Source: CAD feature listing. Evaluate the final solid. Frame: model axes, mm. Face numbers are marked on the shaded views. Give positions to 0.01 mm unless a question says otherwise; leave off trailing zeros. Order: outer loops, then holes, each group sorted by start corner. A loop starts at its lowest first (then second) coordinate and runs counter-clockwise, first axis right, second up. Notation, with made-up numbers: (48.5, -18.75) -> (65.5, -18.75) arc R13 cw to (65.5, -6.75) -> close; hole circle Ø1 at (-19.5, 17). An arc over 180 degrees is marked (long way). Use CSV: the item, a comma, the result in double quotes.
```python
from build123d import *

# Parameters (mm, degrees)
F1_DEPTH = 40.2336
F0_R     = 10.16
F2_DEPTH = 15.7734
F3_R     = 3.302


with BuildPart() as f1:
    # F0 (on Front) → F1 (new body)
    with BuildSketch(Plane.XZ):
        with BuildLine():
            ThreePointArc((9.5121844836, 26.9452959039), (4.8253908933, 28.1646272428), (0, 28.575))
            Line((0, 28.575), (9.5121844836, 26.9452959039))
        make_face()
        with BuildLine():
            Line((9.5121844836, -26.9452959039), (0, -28.575))
            ThreePointArc((0, -28.575), (4.8253908933, -28.1646272428), (9.5121844836, -26.9452959039))
        make_face()
        with BuildLine():
            Line((9.5121844836, 26.9452959039), (0, 28.575))
            ThreePointArc((0, 28.575), (-28.575, 0), (0, -28.575))
            Line((0, -28.575), (9.5121844836, -26.9452959039))
            ThreePointArc((9.5121844836, -26.9452959039), (23.3274655355, -16.5033322905), (28.575, 0))
            ThreePointArc((28.575, 0), (23.3274655355, 16.5033322905), (9.5121844836, 26.9452959039))
        make_face()
        with BuildLine():
            ThreePointArc((-13.4477648793, 4.826), (0, 14.2875), (13.4477648793, 4.826))
            Line((13.4477648793, 4.826), (18.5293, 4.826))
            Line((18.5293, 4.826), (18.5293, -4.826))
            Line((18.5293, -4.826), (13.4477648793, -4.826))
            ThreePointArc((13.4477648793, -4.826), (0, -14.2875), (-13.4477648793, -4.826))
            Line((-13.4477648793, -4.826), (-18.5293, -4.826))
            Line((-18.5293, -4.826), (-18.5293, 4.826))
            Line((-18.5293, 4.826), (-13.4477648793, 4.826))
        make_face(mode=Mode.SUBTRACT)
        with BuildLine():
            ThreePointArc((-13.4477648793, -4.826), (-14.2875, 0), (-13.4477648793, 4.826))
            Line((-13.4477648793, 4.826), (-18.5293, 4.826))
            Line((-18.5293, 4.826), (-18.5293, -4.826))
            Line((-18.5293, -4.826), (-13.4477648793, -4.826))
        make_face()
    extrude(amount=F1_DEPTH)

    # F0 (on Front) → F2 (join)
    with BuildSketch(Plane.XZ):
        with BuildLine():
            Line((9.5121844836, 26.9452959039), (0, 28.575))
            ThreePointArc((0, 28.575), (-28.575, 0), (0, -28.575))
            Line((0, -28.575), (9.5121844836, -26.9452959039))
            ThreePointArc((9.5121844836, -26.9452959039), (23.3274655355, -16.5033322905), (28.575, 0))
            ThreePointArc((28.575, 0), (23.3274655355, 16.5033322905), (9.5121844836, 26.9452959039))
        make_face()
        with BuildLine():
            ThreePointArc((-13.4477648793, 4.826), (0, 14.2875), (13.4477648793, 4.826))
            Line((13.4477648793, 4.826), (18.5293, 4.826))
            Line((18.5293, 4.826), (18.5293, -4.826))
            Line((18.5293, -4.826), (13.4477648793, -4.826))
            ThreePointArc((13.4477648793, -4.826), (0, -14.2875), (-13.4477648793, -4.826))
            Line((-13.4477648793, -4.826), (-18.5293, -4.826))
            Line((-18.5293, -4.826), (-18.5293, 4.826))
            Line((-18.5293, 4.826), (-13.4477648793, 4.826))
        make_face(mode=Mode.SUBTRACT)
        with BuildLine():
            ThreePointArc((9.5121844836, 26.9452959039), (4.8253908933, 28.1646272428), (0, 28.575))
            Line((0, 28.575), (9.5121844836, 26.9452959039))
        make_face()
        with BuildLine():
            Line((9.5121844836, -26.9452959039), (0, -28.575))
            ThreePointArc((0, -28.575), (4.8253908933, -28.1646272428), (9.5121844836, -26.9452959039))
        make_face()
        with BuildLine():
            Line((57.1919272622, 18.7764181619), (9.5121844836, 26.9452959039))
            ThreePointArc((9.5121844836, 26.9452959039), (23.3274655355, 16.5033322905), (28.575, 0))
            ThreePointArc((28.575, 0), (23.3274655355, -16.5033322905), (9.5121844836, -26.9452959039))
            Line((9.5121844836, -26.9452959039), (57.1919272622, -18.7764181619))
            ThreePointArc((57.1919272622, -18.7764181619), (34.925, 0), (57.1919272622, 18.7764181619))
        make_face()
        with BuildLine():
            ThreePointArc((73.025, 0), (68.5383952831, 12.2804730295), (57.1919272622, 18.7764181619))
            ThreePointArc((57.1919272622, 18.7764181619), (34.925, 0), (57.1919272622, -18.7764181619))
            ThreePointArc((57.1919272622, -18.7764181619), (68.5383952831, -12.2804730295), (73.025, 0))
        make_face()
        with Locations((53.975, 0)):
            Circle(F0_R, mode=Mode.SUBTRACT)
    extrude(amount=F2_DEPTH)

    # F3
    f3_edges = [f1.edges().sort_by_distance(p)[0] for p in [
        (0, -40.2336, -28.575),
    ]]
    fillet(f3_edges, radius=F3_R)


solid = f1.part
```
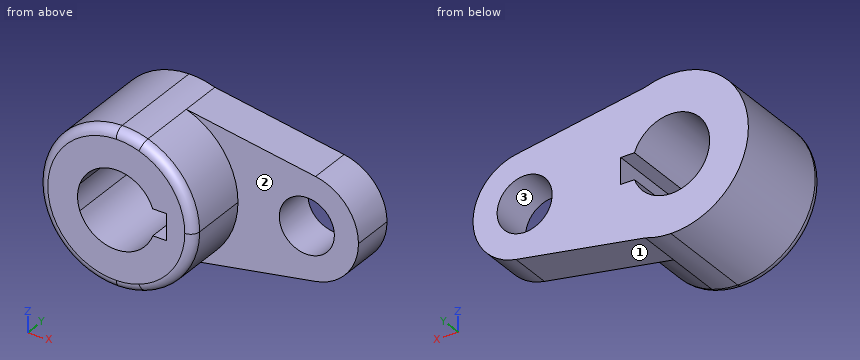
1. Section query C-C on z = -6. Count the separate pieces of the cut face and the enclosed holes in it, plus the area to 3 significant figures.
Answer below:
separate pieces,"3"
enclosed holes,"0"
area,"1,640 mm²"
2. Section query B-B on x = 59.5. Return loops of the section in (y, z).
Answer below:
outline,"(-15.77, -18.23) -> (0, -18.23) -> (0, -8.53) -> (-15.77, -8.53) -> close; (-15.77, 8.53) -> (0, 8.53) -> (0, 18.23) -> (-15.77, 18.23) -> close"
3. Ray query, line 1 along X through (y, z) = (-10, -1.5); line 2 along Z through (x, y) = (7, -24.5); line 3 along Z through (x, y) = (0.5, -37). Return the intervals inside material, ascending.
Answer below:
line 1,"x = -28.54 to -14.21, 18.53 to 43.93, 64.02 to 72.97"
line 2,"z = -27.7 to -12.46, 12.46 to 27.7"
line 3,"z = -28.57 to -14.28, 14.28 to 28.57"
4. Pin query (flat end, axial travel): P1, Ø5.5, axis at x = 16, y = -16, coming from the +Z side; P2, Ø10, axis at x = 37, z = 16, coming from the -Y side; P3, Ø5.5, axis at x = 16, y = -28.5, coming from the -Z side; P4, Ø8, axis at x = 20.5, z = 11.5, coming from the +Y side. Return the tip coordinate at first contact, or that it passes through.
Answer below:
P1,"stops at z = 26.3"
P2,"stops at y = -15.77"
P3,"stops at z = -25.32"
P4,"stops at y = 0"
5. Section query D-D on y = -38. Return loops of the section in (x, z) (1 decimal).
Answer below:
outline,"circle Ø56.8 at (0, 0); hole (13.4, -4.8) -> (18.5, -4.8) -> (18.5, 4.8) -> (13.4, 4.8) arc R14.3 ccw (long way) to start"
6. Mould query, pull axis Z, two halves, no side actions, for the marked faces 1, 2 and 3. Classes: released by +Z, released by -Z, zero draft, split by the parting line, or undercut.
Answer below:
face 1,"released by -Z"
face 2,"zero draft"
face 3,"undercut"
